```python
from build123d import *

# Parameters (mm, degrees)
SKETCH1_R           = 5.08
SKETCH1_R_2         = 12.7
BOSS_EXTRUDE1_DEPTH = 5
SKETCH2_R           = 15.7
SKETCH2_R_2         = 12.7
BOSS_EXTRUDE2_DEPTH = 77.216
SKETCH3_R           = 15.7
BOSS_EXTRUDE3_DEPTH = 3
BOSS_EXTRUDE5_REACH = 64.465
SKETCH4_R           = 6.985
CUT_EXTRUDE1_REACH  = 64.465
SKETCH4_5_R         = 5.08


with BuildPart() as part:
    # Sketch1 → Boss-Extrude1 (new body)
    with BuildSketch(Plane.XY):
        with BuildLine():
            Line((17.630429803, 6.515946667), (8.338716799, 31.656866667))
            ThreePointArc((8.338716799, 31.656866667), (0, 37.465), (-8.338716799, 31.656866667))
            Line((-8.338716799, 31.656866667), (-17.630429803, 6.515946667))
            ThreePointArc((-17.630429803, 6.515946667), (-18.796, 0), (-17.630429803, -6.515946667))
            Line((-17.630429803, -6.515946667), (-8.338716799, -31.656866667))
            ThreePointArc((-8.338716799, -31.656866667), (0, -37.465), (8.338716799, -31.656866667))
            Line((8.338716799, -31.656866667), (17.630429803, -6.515946667))
            ThreePointArc((17.630429803, -6.515946667), (18.796, 0), (17.630429803, 6.515946667))
        make_face()
        with Locations((0, 28.575)):
            Circle(SKETCH1_R, mode=Mode.SUBTRACT)
        Circle(SKETCH1_R_2, mode=Mode.SUBTRACT)
        with Locations((0, -28.575)):
            Circle(SKETCH1_R, mode=Mode.SUBTRACT)
    extrude(amount=BOSS_EXTRUDE1_DEPTH)

    # Sketch2 → Boss-Extrude2 (add)
    with BuildSketch(Plane(origin=(0, 0, 0), x_dir=(-1, 0, 0), z_dir=(0, 0, -1))):
        Circle(SKETCH2_R)
        Circle(SKETCH2_R_2, mode=Mode.SUBTRACT)
    extrude(amount=BOSS_EXTRUDE2_DEPTH)

    # Sketch3 → Boss-Extrude3 (add)
    with BuildSketch(Plane(origin=(0, 0, -77.216), x_dir=(-1, 0, 0), z_dir=(0, 0, -1))):
        Circle(SKETCH3_R)
    extrude(amount=BOSS_EXTRUDE3_DEPTH)

    # Sketch4 → Boss-Extrude5 (add, up to next)
    with BuildSketch(Plane(origin=(0, 25, 0), x_dir=(1, 0, 0), z_dir=(0, 1, 0)), mode=Mode.PRIVATE) as boss_extrude5_sk1:
        with Locations((0, 31.448)):
            Circle(SKETCH4_R)
    boss_extrude5_tool1 = extrude(boss_extrude5_sk1.sketch, amount=-BOSS_EXTRUDE5_REACH, mode=Mode.PRIVATE) - part.part
    add(boss_extrude5_tool1.solids().sort_by_distance((0, 25, -31.448))[0])

    # Sketch4_5 → Cut-Extrude1 (cut, up to next)
    with BuildSketch(Plane(origin=(0, 25, 0), x_dir=(1, 0, 0), z_dir=(0, 1, 0)), mode=Mode.PRIVATE) as cut_extrude1_sk1:
        with Locations((0, 31.448)):
            Circle(SKETCH4_5_R)
    cut_extrude1_tool1 = extrude(cut_extrude1_sk1.sketch, amount=-CUT_EXTRUDE1_REACH, mode=Mode.PRIVATE) & part.part
    add(cut_extrude1_tool1.solids().sort_by_distance((0, 25, -31.448))[0], mode=Mode.SUBTRACT)


solid = part.part
```
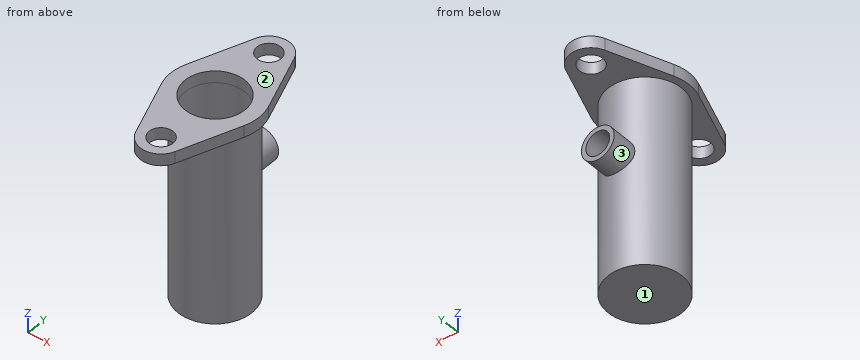
Could you check a few things on this model? Use its own coordinates, in mm. Face numbers are marked on the shaded views. Coordinates: 2 decimals unless noted, no trailing zeros. Write each loop counter-clockwise with the first axis right and the second up, starting at its lowest first coordinate (ties: lowest second). Pieces come first, ordered by that corner, then holes. Notation, with made-up numbers: (45, 62) - (90, 62) arc R6 ccw to (90, 72) - close; hole circle Ø1 at (-32.5, -39). An arc over 180 degrees is marked (long way). Use a Markdown table: item, result.
Q1. Thinking about a two-plate mould opening in Z: for the marked faces 1, 2 and 3, which applies, +Z half, -Z half, draft (parallel to the pull), parting line (faces both ways), or undercut?
Geometry check:
| item | result |
|---|---|
| face 1 | -Z half |
| face 2 | +Z half |
| face 3 | undercut |
Q2. I'm going to push flat-ended pins straight in: pin 1 Ø4 at (y, z) = (-1, -43.5) entering from +X; pin 2 Ø6 at (y, z) = (-17.5, -40.5) entering from -X; pin 3 Ø7 at (x, z) = (-3, -31.5) entering from +Y. Where does each tip first touch, or does it pass through?
Geometry check:
| item | result |
|---|---|
| pin 1 | stops at x = 15.7 |
| pin 2 | stops at x = -6.02 |
| pin 3 | stops at y = 25 |
Q3. Please list where these lines run through material, in increasing order: L1, parallel to X at y = 0, z = 1; L2, parallel to Z at x = -7, y = -2; L3, parallel to Z at x = -12, y = 12.
Geometry check:
| item | result |
|---|---|
| L1 | x = -18.8 to -12.7, 12.7 to 18.8 |
| L2 | z = -80.22 to -77.22 |
| L3 | z = 0 to 5 |
Q4. Imagine slicing it at C-C (y = 0). List the corners of the cut face in (x, z) for me, and give its area (3 significant figures).
Geometry check:
| item | result |
|---|---|
| outline | (-18.8, 0) - (-15.7, 0) - (-15.7, -80.22) - (15.7, -80.22) - (15.7, 0) - (18.8, 0) - (18.8, 5) - (12.7, 5) - (12.7, -77.22) - (-12.7, -77.22) - (-12.7, 5) - (-18.8, 5) - close |
| area | 618 mm2 |
Q5. Imagine slicing it at A-A (x = 0). List the corners of the cut face in (y, z) for me (3 decimals), and give its area (4 significant figures).
Geometry check:
| item | result |
|---|---|
| outline | (-37.465, 0) - (-33.655, 0) - (-33.655, 5) - (-37.465, 5) - close; (-23.495, 0) - (-15.7, 0) - (-15.7, -80.216) - (15.7, -80.216) - (15.7, -38.433) - (25, -38.433) - (25, -36.528) - (12.7, -36.528) - (12.7, -77.216) - (-12.7, -77.216) - (-12.7, 5) - (-23.495, 5) - close; (12.7, -26.368) - (25, -26.368) - (25, -24.463) - (15.7, -24.463) - (15.7, 0) - (23.495, 0) - (23.495, 5) - (12.7, 5) - close; (33.655, 0) - (37.465, 0) - (37.465, 5) - (33.655, 5) - close |
| area | 708.5 mm2 |
Q6. Imagine slicing it at B-B (y = 20). List the corners of the cut face in (x, z) for me (3 decimals), and give its area (3 significant figures).
Geometry check:
| item | result |
|---|---|
| outline | (-12.647, 0) - (12.647, 0) - (12.647, 5) - (-12.647, 5) - close; circle Ø13.97 at (0, -31.448); hole circle Ø10.16 at (0, -31.448) |
| area | 199 mm2 |
Q7. Imagine slicing it at D-D (y = -27). List the corners of the cut face in (x, z) for me, and give its area (3 significant figures).
Geometry check:
| item | result |
|---|---|
| outline | (-10.06, 0) - (-4.83, 0) - (-4.83, 5) - (-10.06, 5) - close; (4.83, 0) - (10.06, 0) - (10.06, 5) - (4.83, 5) - close |
| area | 52.3 mm2 |
